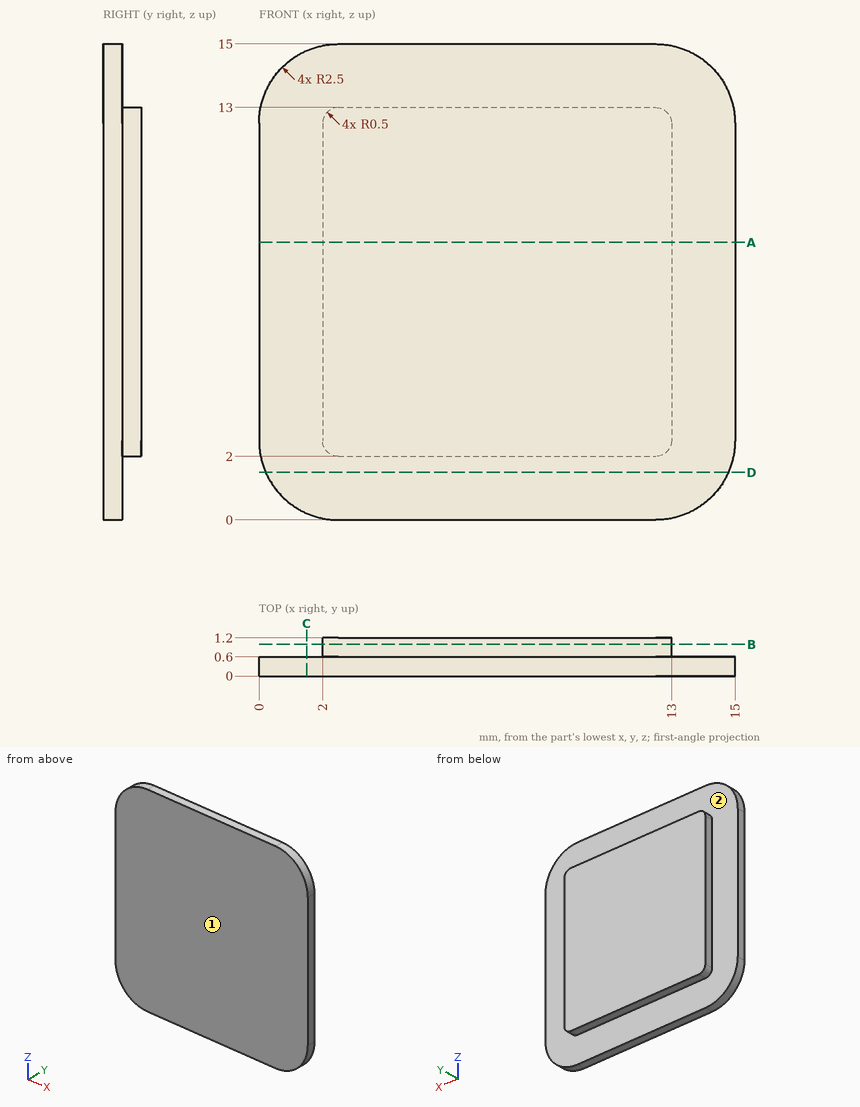
Input: dimensioned drawing with shaded views. Units: mm. Origin: part minimum x, y, z. A direction names the side the tool comes from. Round coordinates to 2 decimals unless told otherwise and drop trailing zeros. Loops run counter-clockwise (first coordinate to the right, second up) from the corner with the lowest first, then second, coordinate; pieces in that order, holes last. Notation, with made-up numbers: (85.5, 56.25) -> (114.5, 56.25) arc R24 cw to (114.5, 84.25) -> close; hole circle Ø1 at (5, 41.25). An arc over 180 degrees is marked (long way). Use one line per item in the form item = value. Start each with the question number.
1) Section D-D on z = 1.5. Output: boundary loops of the cut face in (x, y).
2) Access query for the marked faces 1 and 2. Directions: +Z, -Z, +X, -X, +Y, -Y. A direction counts if a zero-diameter tool reaches every point of the face in a straight line with its end or side. Return the directions, or none.
3) Section B-B on y = 1. Output: boundary loops of the cut face in (x, z).
4) Section C-C on x = 1.5. Output: boundary loops of the cut face in (y, z), then the cut area to 3 significant figures.
5) First-contact query: P1, Ø0.7, axis at y = 1, z = 5, coming from the -X side; P2, Ø0.5, axis at y = 1, z = 6, coming from the +X side; P3, Ø4, axis at x = 6, z = 10, coming from the -Y side; P4, Ø0.5, axis at x = 9.5, y = 1, coming from the -Z side. Flat tips, straight axial feed; report the tip coordinate or a pass-through.
6) Line query: L1, parallel to X at y = 0.7, z = 9; L2, parallel to X at y = 0.55, z = 12.75. Output: solid intervals per line, ascending.
7) Section A-A on z = 8.75. Output: boundary loops of the cut face in (x, y), then the cut area to 3 significant figures.
Response:
q1.outline = (0.21, 0) -> (14.79, 0) -> (14.79, 0.6) -> (0.21, 0.6) -> close
q2.face_1 = +Z, -Z, +X, -X, -Y
q2.face_2 = +Y
q3.outline = (2, 2.5) arc R0.5 ccw to (2.5, 2) -> (12.5, 2) arc R0.5 ccw to (13, 2.5) -> (13, 12.5) arc R0.5 ccw to (12.5, 13) -> (2.5, 13) arc R0.5 ccw to (2, 12.5) -> close
q4.outline = (0, 0.21) -> (0.6, 0.21) -> (0.6, 14.79) -> (0, 14.79) -> close
q4.area = 8.75 mm^2
q5.P1 = 2
q5.P2 = 13
q5.P3 = 0
q5.P4 = 2
q6.L1 = 2 to 13
q6.L2 = 0.01 to 14.99
q7.outline = (0, 0) -> (15, 0) -> (15, 0.6) -> (13, 0.6) -> (13, 1.2) -> (2, 1.2) -> (2, 0.6) -> (0, 0.6) -> close
q7.area = 15.6 mm^2
